Answer from the drawing. Dimensions are ordinates in mm from the lowest x, y and z of the part. Coordinates: 2 decimals unless noted, no trailing zeros. Loops run counter-clockwise (first coordinate to the right, second up) from the corner with the lowest first, then second, coordinate; pieces in that order, holes last. Notation, with made-up numbers: (-28, 3) - (5, 3) arc R25 ccw to (5, 39) - close; hole circle Ø8 at (86, -24.75). An arc over 180 degrees is marked (long way). Write each question's results on one line, items separated by ' | '. Start each with the question number.
1. This flat-tipped pin is pushed along its axis until it touches: P1, Ø3, axis at y = 7.5, z = 3.5, coming from the -X side. Where does it stop, or does it pass through?
2. A cutting plane is placed at A-A on x = 12. Determine the outline of the cut face in (y, z).
3. A cutting plane is placed at C-C on z = 9. Determine the outline of the cut face in (x, y).
4. Find the intervals of material crossed by line 1 along Y through (x, z) = (12, 6); line 2 along Y through (x, z) = (11, 9.5); line 3 along X through (y, z) = (21, 6.5), in increasing order. Write a range as [from, to].
5. A cutting plane is placed at B-B on y = 12. Determine the outline of the cut face in (x, z), then the cut area to 4 significant figures.
6. Determine the mould class of the marked faces 1, 2 and 3 for opening direction Y: released by +Y, released by -Y, zero draft, split by the parting line, or undercut.
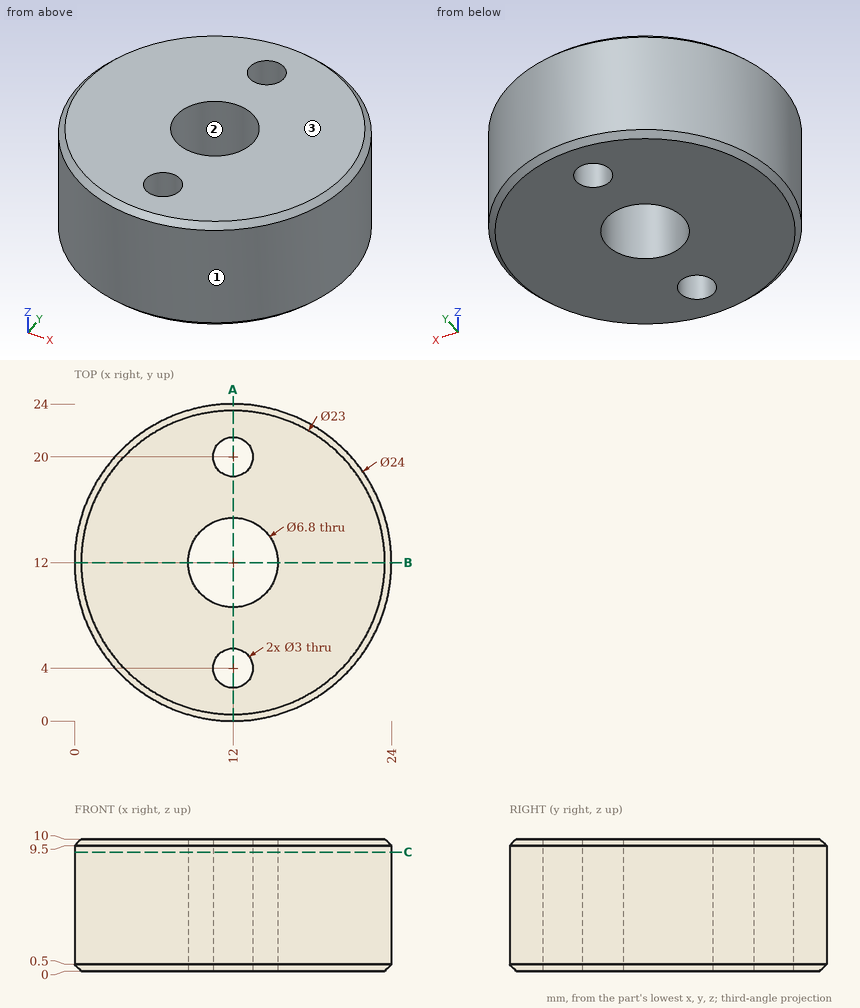
Values:
1) P1: x = 0.38
2) outline: (0, 0.5) - (0.5, 0) - (2.5, 0) - (2.5, 10) - (0.5, 10) - (0, 9.5) - close; (5.5, 0) - (8.6, 0) - (8.6, 10) - (5.5, 10) - close; (15.4, 0) - (18.5, 0) - (18.5, 10) - (15.4, 10) - close; (21.5, 0) - (23.5, 0) - (24, 0.5) - (24, 9.5) - (23.5, 10) - (21.5, 10) - close
3) outline: circle Ø24 at (12, 12); hole circle Ø6.8 at (12, 12); hole circle Ø3 at (12, 4); hole circle Ø3 at (12, 20)
4) line 1: [0, 2.5], [5.5, 8.6], [15.4, 18.5], [21.5, 24] | line 2: [0.04, 2.88], [5.12, 8.75], [15.25, 18.88], [21.12, 23.96] | line 3: [4.06, 10.88], [13.12, 19.94]
5) outline: (0, 0.5) - (0.5, 0) - (8.6, 0) - (8.6, 10) - (0.5, 10) - (0, 9.5) - close; (15.4, 0) - (23.5, 0) - (24, 0.5) - (24, 9.5) - (23.5, 10) - (15.4, 10) - close | area: 171.5 mm^2
6) face 1: split by the parting line | face 2: undercut | face 3: zero draft
